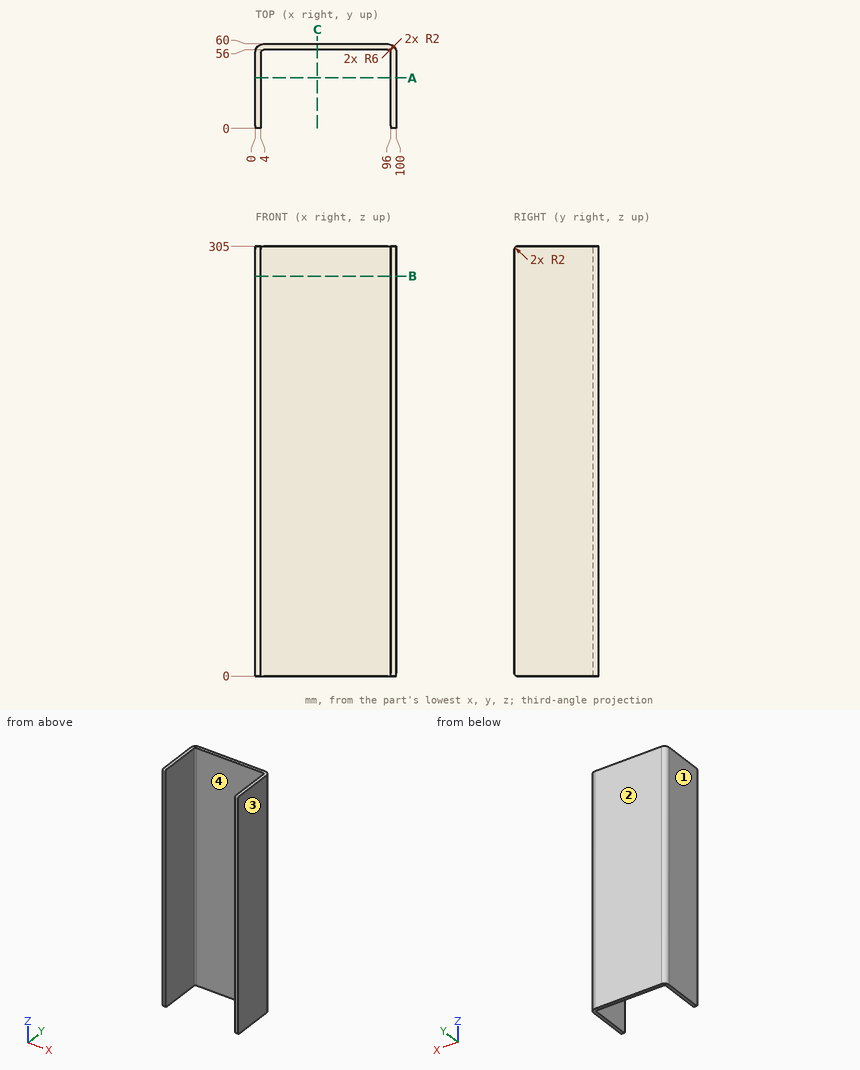
Part print with two shaded views. Sizes in mm from the minimum x, y, z corner. Coordinates: 2 decimals unless noted, no trailing zeros. Write each loop counter-clockwise with the first axis right and the second up, starting at its lowest first coordinate (ties: lowest second). Pieces come first, ordered by that corner, then holes. Notation, with made-up numbers: M 57.25,10 L 71.25,10 A19 ccw 71.25,16 Z; hole C 2,-30 d9. An arc over 180 degrees is marked long. Return JSON: item names as keys, results as strings.
Item 1: Probe line 1 (X direction, y = 32.5, z = 114.5); line 2 (Y direction, x = 46, z = 110.5); line 3 (Y direction, x = 5, z = 252). List the from-to ranges inside material, lowest first. Write a range as from..to.
Findings below:
{"line 1": "x = 0..4, 96..100", "line 2": "y = 56..60", "line 3": "y = 55.73..59.92"}
Item 2: Slice it at C-C, the plane x = 44. Write the cut outline in (y, z).
Findings below:
{"outline": "M 56,0 L 60,0 L 60,305 L 56,305 Z"}
Item 3: Slice it at A-A, the plane y = 36. Write the cut outline in (x, z).
Findings below:
{"outline": "M 0,0 L 4,0 L 4,305 L 0,305 Z; M 96,0 L 100,0 L 100,305 L 96,305 Z"}
Item 4: Slice it at B-B, the plane z = 284. Write the cut outline in (x, y), and give its area (3 significant figures).
Findings below:
{"outline": "M 0,0 L 4,0 L 4,54 A2 cw 6,56 L 94,56 A2 cw 96,54 L 96,0 L 100,0 L 100,54 A6 ccw 94,60 L 6,60 A6 ccw 0,54 Z", "area": "834 mm2"}
Item 5: Two-plate mould, pull along X, no slides. Class the marked faces 1, 2, 3 and 4: +X half, -X half, draft (parallel to the pull), parting line (faces both ways), or undercut.
Findings below:
{"face 1": "-X half", "face 2": "draft", "face 3": "+X half", "face 4": "undercut"}
Item 6: Drop a flat-ended pin along its axis: pin 1 Ø4 at (x, z) = (88, 60.5) entering from -Y. Give the stop position or say it passes through.
Findings below:
{"pin 1": "stops at y = 56"}
